The model under review builds one solid part; all positions refer to its coordinate system, in mm. A direction names the side the tool comes from. Give positions to 0.01 mm unless a question says otherwise; leave off trailing zeros. Write each loop counter-clockwise with the first axis right and the second up, starting at its lowest first coordinate (ties: lowest second). Pieces come first, ordered by that corner, then holes. Notation, with made-up numbers: (46, 6) -> (80, 6) arc R14 ccw to (80, 12) -> close; hole circle Ø10 at (-8.75, 71). An arc over 180 degrees is marked (long way). Use CSV: the item, a comma, the result in double quotes.
```python
from build123d import *

# Parameters (mm, degrees)
SKETCH004_R     = 1.7
PAD002_DEPTH    = 2
SKETCH005_W     = 4
SKETCH005_H     = 8
PAD003_DEPTH    = 9.8
SKETCH006_R     = 2.35
POCKET001_DEPTH = 5
FILLET001_R     = 4.8


with BuildPart() as part:
    # Sketch004 (on DatumPlane) → Pad002 (new body)
    with BuildSketch(Plane.YZ.offset(2)):
        with BuildLine():
            ThreePointArc((-7, -9.9), (-2.1, -5), (-7, -0.1))
            Line((-7, -0.1), (-20, -0.1))
            Line((-20, -0.1), (-20, -9.9))
            Line((-20, -9.9), (-7, -9.9))
        make_face()
        with Locations((-7, -5)):
            Circle(SKETCH004_R, mode=Mode.SUBTRACT)
    extrude(amount=PAD002_DEPTH)

    # Sketch005 (on Face4 of Pad002) → Pad003 (join)
    with BuildSketch(Plane(origin=(2, 0, -9.9), x_dir=(0, 1, 0), z_dir=(0, 0, -1))):
        with Locations((-18, 6)):
            Rectangle(SKETCH005_W, SKETCH005_H)
    extrude(amount=-PAD003_DEPTH)

    # Sketch006 (on Face9 of Pad003) → Pocket001 (cut)
    with BuildSketch(Plane(origin=(2, -20, 0), x_dir=(0, 0, -1), z_dir=(0, -1, 0))):
        with Locations((5, 5)):
            Circle(SKETCH006_R)
    extrude(amount=-POCKET001_DEPTH, mode=Mode.SUBTRACT)

    # Fillet001
    fillet001_edges = [part.edges().sort_by_distance(p)[0] for p in [
        (12, -18, -0.1),
        (12, -18, -9.9),
    ]]
    fillet(fillet001_edges, radius=FILLET001_R)


solid = part.part
```
Q1. Consider section D-D (z = -2.25). Write out the cut boundary in (x, y), then the cut area to 3 significant figures.
Derived:
outline,"(2, -20) -> (11.2, -20) -> (11.2, -16) -> (4, -16) -> (4, -2.94) -> (2, -2.94) -> close"
area,"62.9 mm2"
Q2. Consider section C-C (y = -7.5). Write out the cut boundary in (x, z), then the cut area to 3 significant figures.
Derived:
outline,"(2, -9.9) -> (4, -9.9) -> (4, -6.62) -> (2, -6.62) -> close; (2, -3.38) -> (4, -3.38) -> (4, -0.1) -> (2, -0.1) -> close"
area,"13.1 mm2"
Q3. Consider section B-B (z = -4). Write out the cut boundary in (x, y).
Derived:
outline,"(2, -20) -> (4.87, -20) -> (4.87, -16) -> (4, -16) -> (4, -8.37) -> (2, -8.37) -> close; (2, -5.63) -> (4, -5.63) -> (4, -2.2) -> (2, -2.2) -> close; (9.13, -20) -> (11.91, -20) -> (11.91, -16) -> (9.13, -16) -> close"
Q4. Insertion check: pin 1 (4 mm diameter, centred on y = -11.5, z = -2.5, fed in from +X); pin 2 (2 mm diameter, centred on y = -7, z = -5, fed in from +X); pin 3 (4 mm diameter, centred on x = 9, z = -5.5, fed in from +Y). Each pin has a flat end and moves straight along its axis. Give the tip position at first contact, or say it passes through.
Derived:
pin 1,"stops at x = 4"
pin 2,"passes through"
pin 3,"stops at y = -16"
Q5. Consider section A-A (y = -18). Write out the cut boundary in (x, z), then the cut area to 3 significant figures.
Derived:
outline,"(2, -9.9) -> (7.2, -9.9) arc R4.8 ccw to (12, -5.1) -> (12, -4.9) arc R4.8 ccw to (7.2, -0.1) -> (2, -0.1) -> close; hole circle Ø4.7 at (7, -5)"
area,"70.8 mm2"
Q6. To check wall thickness, follow probe 1 along Z at (x, y) = (3.1, -7); probe 2 along X at (y, z) = (-18.9, -5); probe 3 along X at (y, z) = (-15.75, -9). State the ranges of each line that lie inside material, in increasing order.
Derived:
probe 1,"z = -9.9 to -6.7, -3.3 to -0.1"
probe 2,"x = 2 to 4.65, 9.35 to 12"
probe 3,"x = 2 to 4"
Q7. Machinability: for faces 1 (the flat face through (4, -9, -5)), 2 (the cylindrical face through (10.63, -17.97, -1.54)), which of the approach directions +Z, -Z, +X, -X, +Y, -Y give a long, thin tool a straight path to every point of the face, cutting with its end or side? Answer none if there is none.
Derived:
face 1,"+Z, -Z, +X, +Y"
face 2,"+Z, +X, +Y, -Y"
Q8. The part is to be moulded in two halves that separate along Z. For faces 3 (the flat face through (10, -16, -5)), 4 (the cylindrical face through (4.915, -18.028, -6.084)), 5 (the cylindrical face through (2.99, -7.37, -6.66)), 6 (the cylindrical face through (3, -2.1, -5.1)), say which applies: pulls with the +Z half, pulls with the -Z half, needs draft (parallel to the pull), parting line crosses it, or undercut.
Derived:
face 3,"needs draft"
face 4,"undercut"
face 5,"undercut"
face 6,"parting line crosses it"
